Can you work these out from the model? Positions are in its coordinate system, mm. Face numbers are marked on the shaded views. A direction names the side the tool comes from. Round coordinates to 2 decimals unless told otherwise and drop trailing zeros. Write each loop counter-clockwise with the first axis right and the second up, starting at its lowest first coordinate (ties: lowest second). Pieces come first, ordered by that corner, then holes. Notation, with made-up numbers: M 29,64.25 L 69,64.25 A7 cw 69,69.25 Z; hole C 43,52 d2. An arc over 180 degrees is marked long. Answer in a Markdown table with one row per item. Add a question column.
(1) If we mould it in two halves opening along X, with no side actions, what happens to the marked faces 1, 2, 3 and 4? For each: released by +X, released by -X, zero draft, split by the parting line, or undercut.
(2) Suppose I cut it at A-A, the plane x = 0. Write out the boundary of the cut face in (y, z), then the cut area to 3 significant figures.
(3) If I drill on probe 1 along Y at (x, z) = (12, -20.5); probe 2 along Z at (x, y) = (-22, -48); probe 3 along X at (y, z) = (-17.5, -28), over which ranges is the centre line in solid material (lowest first)?
(4) I'm going to push flat-ended pins straight in: pin 1 (5 mm diameter, centred on x = 14.5, z = 33.5, fed in from -Y); pin 2 (3.5 mm diameter, centred on x = -24, y = -28.5, fed in from +Z); pin 3 (8.5 mm diameter, centred on y = -28.5, z = -36, fed in from +X). Where does each tip first touch, or does it pass through?
(5) Suppose I cut it at D-D, the plane z = -14. Write out the boundary of the cut face in (x, y).
(6) Suppose I cut it at C-C, the plane x = 17.5. Write out the boundary of the cut face in (y, z).
(7) Suppose I cut it at B-B, the plane z = 24.5. Write out the boundary of the cut face in (x, y).
(8) For the marked faces 5, 6 and 7, which set-ups out of +Z, -Z, +X, -X, +Y, -Y let a thin tool reach every point of the face, with its end or its side?
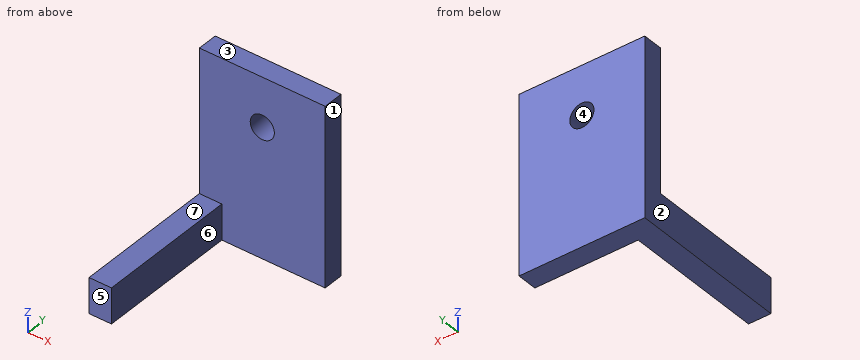
from build123d import *

# Parameters (mm, degrees)
SKETCH1_W           = 62.2
SKETCH1_H           = 88.01
BOSS_EXTRUDE1_DEPTH = 10
SKETCH2_R           = 5.969
CUT_EXTRUDE1_DEPTH  = 10
SKETCH3_W           = 11.09
SKETCH3_H           = 17.48264
BOSS_EXTRUDE2_DEPTH = 69.9


with BuildPart() as part:
    # Sketch1 → Boss-Extrude1 (new body)
    with BuildSketch(Plane(origin=(0, 0, 0), x_dir=(1, 0, 0), z_dir=(0, 1, 0))):
        with Locations((0, -3.512935)):
            Rectangle(SKETCH1_W, SKETCH1_H)
    extrude(amount=BOSS_EXTRUDE1_DEPTH)

    # Sketch2 → Cut-Extrude1 (cut)
    with BuildSketch(Plane(origin=(0, 10, 0), x_dir=(1, 0, 0), z_dir=(0, 1, 0))):
        with Locations(Location((0, -23.217935, 0), (0, 0, 270))):
            Circle(SKETCH2_R)
    extrude(amount=-CUT_EXTRUDE1_DEPTH, mode=Mode.SUBTRACT)

    # Sketch3 → Boss-Extrude2 (add)
    with BuildSketch(Plane.XZ):
        with Locations((-25.555, -31.750745)):
            Rectangle(SKETCH3_W, SKETCH3_H)
    extrude(amount=BOSS_EXTRUDE2_DEPTH)


solid = part.part
Calculated:
| question | item | result |
|---|---|---|
| 1 | face 1 | released by +X |
| 1 | face 2 | released by -X |
| 1 | face 3 | zero draft |
| 1 | face 4 | undercut |
| 2 | outline | M 0,-40.49 L 10,-40.49 L 10,17.25 L 0,17.25 Z; M 0,29.19 L 10,29.19 L 10,47.52 L 0,47.52 Z |
| 2 | area | 761 mm² |
| 3 | probe 1 | 0 to 10 |
| 3 | probe 2 | -40.49 to -23.01 |
| 3 | probe 3 | -31.1 to -20.01 |
| 4 | pin 1 | y = 0 |
| 4 | pin 2 | z = -23.01 |
| 4 | pin 3 | x = -20.01 |
| 5 | outline | M -31.1,0 L 31.1,0 L 31.1,10 L -31.1,10 Z |
| 6 | outline | M 0,-40.49 L 10,-40.49 L 10,47.52 L 0,47.52 Z |
| 7 | outline | M -31.1,0 L -5.83,0 L -5.83,10 L -31.1,10 Z; M 5.83,0 L 31.1,0 L 31.1,10 L 5.83,10 Z |
| 8 | face 5 | +Z, -Z, +X, -X, -Y |
| 8 | face 6 | +Z, -Z, +X, -Y |
| 8 | face 7 | +Z, +X, -X, -Y |
